Could you check a few things on this model? Use its own coordinates, in mm. Coordinates: 2 decimals unless noted, no trailing zeros. Write each loop counter-clockwise with the first axis right and the second up, starting at its lowest first coordinate (ties: lowest second). Pieces come first, ordered by that corner, then holes. Notation, with made-up numbers: M 68,81 L 113,81 A20 cw 113,96 Z; hole C 53.25,-10.5 d8. An arc over 180 degrees is marked long. Write item = value, one per line.
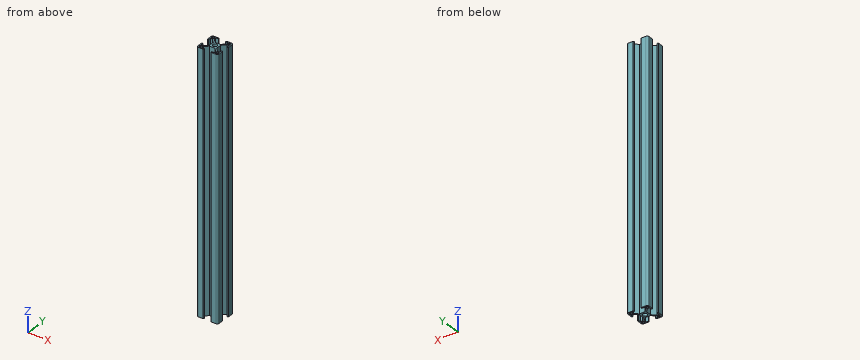
```python
from build123d import *

# Parameters (mm, degrees)
CROQUIS1_R              = 3.4
SALIENTE_EXTRUIR1_DEPTH = 400


with BuildPart() as part:
    # Croquis1 → Saliente-Extruir1 (new body)
    with BuildSketch(Plane.XY):
        with BuildLine():
            Line((5.8, -4.24), (5.8, 4.24))
            Line((5.8, 4.24), (11.47, 9.91))
            Line((11.47, 9.91), (14.66, 9.91))
            Line((14.66, 9.91), (14.66, 5.73))
            Line((14.66, 5.73), (15.66, 5.73))
            ThreePointArc((15.66, 5.73), (16.367106781, 6.022893219), (16.66, 6.73))
            Line((16.66, 6.73), (16.66, 14.16))
            ThreePointArc((16.66, 14.16), (15.927766953, 15.927766953), (14.16, 16.66))
            Line((14.16, 16.66), (6.73, 16.66))
            ThreePointArc((6.73, 16.66), (6.022893219, 16.367106781), (5.73, 15.66))
            Line((5.73, 15.66), (5.73, 14.66))
            Line((5.73, 14.66), (9.91, 14.66))
            Line((9.91, 14.66), (9.91, 11.47))
            Line((9.91, 11.47), (4.24, 5.8))
            Line((4.24, 5.8), (-4.24, 5.8))
            Line((-4.24, 5.8), (-9.91, 11.47))
            Line((-9.91, 11.47), (-9.91, 14.66))
            Line((-9.91, 14.66), (-5.73, 14.66))
            Line((-5.73, 14.66), (-5.73, 15.66))
            ThreePointArc((-5.73, 15.66), (-6.022893219, 16.367106781), (-6.73, 16.66))
            Line((-6.73, 16.66), (-14.16, 16.66))
            ThreePointArc((-14.16, 16.66), (-15.927766953, 15.927766953), (-16.66, 14.16))
            Line((-16.66, 14.16), (-16.66, 6.73))
            ThreePointArc((-16.66, 6.73), (-16.367106781, 6.022893219), (-15.66, 5.73))
            Line((-15.66, 5.73), (-14.66, 5.73))
            Line((-14.66, 5.73), (-14.66, 9.91))
            Line((-14.66, 9.91), (-11.47, 9.91))
            Line((-11.47, 9.91), (-5.8, 4.24))
            Line((-5.8, 4.24), (-5.8, -4.24))
            Line((-5.8, -4.24), (-11.47, -9.91))
            Line((-11.47, -9.91), (-14.66, -9.91))
            Line((-14.66, -9.91), (-14.66, -5.73))
            Line((-14.66, -5.73), (-15.66, -5.73))
            ThreePointArc((-15.66, -5.73), (-16.367106781, -6.022893219), (-16.66, -6.73))
            Line((-16.66, -6.73), (-16.66, -14.16))
            ThreePointArc((-16.66, -14.16), (-15.927766953, -15.927766953), (-14.16, -16.66))
            Line((-14.16, -16.66), (-6.73, -16.66))
            ThreePointArc((-6.73, -16.66), (-6.022893219, -16.367106781), (-5.73, -15.66))
            Line((-5.73, -15.66), (-5.73, -14.66))
            Line((-5.73, -14.66), (-9.91, -14.66))
            Line((-9.91, -14.66), (-9.91, -11.47))
            Line((-9.91, -11.47), (-4.24, -5.8))
            Line((-4.24, -5.8), (4.24, -5.8))
            Line((4.24, -5.8), (9.91, -11.47))
            Line((9.91, -11.47), (9.91, -14.66))
            Line((9.91, -14.66), (5.73, -14.66))
            Line((5.73, -14.66), (5.73, -15.66))
            ThreePointArc((5.73, -15.66), (6.022893219, -16.367106781), (6.73, -16.66))
            Line((6.73, -16.66), (14.16, -16.66))
            ThreePointArc((14.16, -16.66), (15.927766953, -15.927766953), (16.66, -14.16))
            Line((16.66, -14.16), (16.66, -6.73))
            ThreePointArc((16.66, -6.73), (16.367106781, -6.022893219), (15.66, -5.73))
            Line((15.66, -5.73), (14.66, -5.73))
            Line((14.66, -5.73), (14.66, -9.91))
            Line((14.66, -9.91), (11.47, -9.91))
            Line((11.47, -9.91), (5.8, -4.24))
        make_face()
        Circle(CROQUIS1_R, mode=Mode.SUBTRACT)
        with BuildLine():
            Line((11.651495134, 14.901495134), (14.401495134, 14.901495134))
            ThreePointArc((14.401495134, 14.901495134), (14.755048524, 14.755048524), (14.901495134, 14.401495134))
            Line((14.901495134, 14.401495134), (14.901495134, 11.651495134))
            ThreePointArc((14.901495134, 11.651495134), (14.755048524, 11.297941743), (14.401495134, 11.151495134))
            Line((14.401495134, 11.151495134), (11.651495134, 11.151495134))
            ThreePointArc((11.651495134, 11.151495134), (11.297941743, 11.297941743), (11.151495134, 11.651495134))
            Line((11.151495134, 11.651495134), (11.151495134, 14.401495134))
            ThreePointArc((11.151495134, 14.401495134), (11.297941743, 14.755048524), (11.651495134, 14.901495134))
        make_face(mode=Mode.SUBTRACT)
        with BuildLine():
            Line((-14.901495134, 14.401495134), (-14.901495134, 11.651495134))
            ThreePointArc((-14.901495134, 11.651495134), (-14.755048524, 11.297941743), (-14.401495134, 11.151495134))
            Line((-14.401495134, 11.151495134), (-11.651495134, 11.151495134))
            ThreePointArc((-11.651495134, 11.151495134), (-11.297941743, 11.297941743), (-11.151495134, 11.651495134))
            Line((-11.151495134, 11.651495134), (-11.151495134, 14.401495134))
            ThreePointArc((-11.151495134, 14.401495134), (-11.297941743, 14.755048524), (-11.651495134, 14.901495134))
            Line((-11.651495134, 14.901495134), (-14.401495134, 14.901495134))
            ThreePointArc((-14.401495134, 14.901495134), (-14.755048524, 14.755048524), (-14.901495134, 14.401495134))
        make_face(mode=Mode.SUBTRACT)
        with BuildLine():
            Line((-11.651495134, -14.901495134), (-14.401495134, -14.901495134))
            ThreePointArc((-14.401495134, -14.901495134), (-14.755048524, -14.755048524), (-14.901495134, -14.401495134))
            Line((-14.901495134, -14.401495134), (-14.901495134, -11.651495134))
            ThreePointArc((-14.901495134, -11.651495134), (-14.755048524, -11.297941743), (-14.401495134, -11.151495134))
            Line((-14.401495134, -11.151495134), (-11.651495134, -11.151495134))
            ThreePointArc((-11.651495134, -11.151495134), (-11.297941743, -11.297941743), (-11.151495134, -11.651495134))
            Line((-11.151495134, -11.651495134), (-11.151495134, -14.401495134))
            ThreePointArc((-11.151495134, -14.401495134), (-11.297941743, -14.755048524), (-11.651495134, -14.901495134))
        make_face(mode=Mode.SUBTRACT)
        with BuildLine():
            Line((14.901495134, -14.401495134), (14.901495134, -11.651495134))
            ThreePointArc((14.901495134, -11.651495134), (14.755048524, -11.297941743), (14.401495134, -11.151495134))
            Line((14.401495134, -11.151495134), (11.651495134, -11.151495134))
            ThreePointArc((11.651495134, -11.151495134), (11.297941743, -11.297941743), (11.151495134, -11.651495134))
            Line((11.151495134, -11.651495134), (11.151495134, -14.401495134))
            ThreePointArc((11.151495134, -14.401495134), (11.297941743, -14.755048524), (11.651495134, -14.901495134))
            Line((11.651495134, -14.901495134), (14.401495134, -14.901495134))
            ThreePointArc((14.401495134, -14.901495134), (14.755048524, -14.755048524), (14.901495134, -14.401495134))
        make_face(mode=Mode.SUBTRACT)
    extrude(amount=SALIENTE_EXTRUIR1_DEPTH)


solid = part.part
```
Item 1: Imagine slicing it at A-A (y = 0). Write out the boundary of the cut face in (x, z).
Numbers:
outline = M -5.8,0 L -3.4,0 L -3.4,400 L -5.8,400 Z; M 3.4,0 L 5.8,0 L 5.8,400 L 3.4,400 Z
Item 2: Imagine slicing it at C-C (z = 132). State how many separate pieces and enclosed holes the cut face has, and give its area (3 significant figures).
Numbers:
separate_pieces = 1
enclosed_holes = 5
area = 346 mm²
Item 3: I'm going to push flat-ended pins straight in: P1, Ø6, axis at x = -2, z = 260, coming from the +Y side; P2, Ø2.5, axis at y = 1.5, z = 277, coming from the -X side; P3, Ø9.5, axis at y = 0, z = 110.5, coming from the +X side. Where does each tip first touch, or does it pass through?
Numbers:
P1 = 6.56
P2 = -5.8
P3 = 6.31
Item 4: If I drill on line 1 along Y through (x, z) = (13, 105.5); line 2 along Y through (x, z) = (9, 106), over which ranges is the centre line in solid material (lowest first)?
Numbers:
line_1 = -16.66 to -14.9, -11.15 to -9.91, 9.91 to 11.15, 14.9 to 16.66
line_2 = -16.66 to -14.66, -10.56 to -7.44, 7.44 to 10.56, 14.66 to 16.66
